Verification items for the finished model (mm, model axes). A direction names the side the tool comes from. Round coordinates to 2 decimals unless told otherwise and drop trailing zeros. Loops run counter-clockwise (first coordinate to the right, second up) from the corner with the lowest first, then second, coordinate; pieces in that order, holes last. Notation, with made-up numbers: (49, 37) -> (60, 37) arc R35 cw to (60, 73) -> close; hole circle Ø9 at (-29, 16). An arc over 180 degrees is marked (long way). Write item = value, one per line.
```python
from build123d import *

# Parameters (mm, degrees)
SKETCH_1_W             = 70
SKETCH_1_H             = 43
EXTRUDE_1_DEPTH        = 10
SKETCH_8_W             = 24.88
SKETCH_8_H             = 5
CUT_EXTRUDE_4_DEPTH    = 57.338264084
EXTRUDE_1_2_DEPTH      = 5
EXTRUDE_1_2_DEPTH_BACK = 2
SKETCH_11_R            = 20.45
SKETCH_11_R_2          = 12.45
CUT_EXTRUDE_6_DEPTH    = 5
CUT_EXTRUDE_7_DEPTH    = 5
SKETCH_16_W            = 5.88
SKETCH_16_H            = 11
CUT_EXTRUDE_8_DEPTH    = 5
SKETCH_17_W            = 5.88
SKETCH_17_H            = 8.352111755
CUT_EXTRUDE_9_DEPTH    = 5
CUT_EXTRUDE_10_DEPTH   = 5
CUT_EXTRUDE_11_DEPTH   = 5
SKETCH_21_R            = 3
CUT_EXTRUDE_12_DEPTH   = 43.275879648
SKETCH_22_R            = 3
CUT_EXTRUDE_13_DEPTH   = 43.275879648
SKETCH_24_R            = 3.51
CUT_EXTRUDE_15_DEPTH   = 7
SKETCH_27_W            = 5.88
SKETCH_27_H            = 8.139673367
CUT_EXTRUDE_16_DEPTH   = 7
SKETCH_31_W            = 6.88
SKETCH_31_H            = 8.484679277
CUT_EXTRUDE_21_DEPTH   = 14.5
CUT_EXTRUDE_22_DEPTH   = 42.379342672
CUT_EXTRUDE_23_DEPTH   = 42.379342672
CUT_EXTRUDE_24_DEPTH   = 42.379342672
CUT_EXTRUDE_25_DEPTH   = 14.5
CUT_EXTRUDE_26_DEPTH   = 14.5
CUT_EXTRUDE_27_DEPTH   = 14.5
FILLET_1_R             = 10


with BuildPart() as part:
    # 草圖1 → Extrude 1 (new body)
    with BuildSketch(Plane(origin=(0, 0, 0), x_dir=(1, 0, 0), z_dir=(0, 1, 0))):
        Rectangle(SKETCH_1_W, SKETCH_1_H)
    extrude(amount=EXTRUDE_1_DEPTH)

    # 草圖8 → 除料-伸長4 (cut, through all)
    with BuildSketch(Plane.XY.offset(21.5)):
        with Locations((0.06, 7.5)):
            Rectangle(SKETCH_8_W, SKETCH_8_H)
    extrude(amount=-CUT_EXTRUDE_4_DEPTH, mode=Mode.SUBTRACT)

    # 草圖11 → Extrude 1 2 (add, two sides: drawn at the far end of the back side and taken through both)
    with BuildSketch(Plane(origin=(0, 5, 0), x_dir=(1, 0, 0), z_dir=(0, 1, 0)).offset(-EXTRUDE_1_2_DEPTH_BACK)):
        with Locations((0.06, 0)):
            Circle(SKETCH_11_R)
        with Locations((0.06, 0)):
            Circle(SKETCH_11_R_2, mode=Mode.SUBTRACT)
    extrude(amount=EXTRUDE_1_2_DEPTH + EXTRUDE_1_2_DEPTH_BACK)

    # 草圖14 → 除料-伸長6 (cut)
    with BuildSketch(Plane(origin=(0, 5, 0), x_dir=(1, 0, 0), z_dir=(0, 1, 0))):
        Polygon((0.06, -20.45), (12.5, -20.45), (12.5, -21.5), (-12.38, -21.5), (-12.38, -20.45), align=None)
    extrude(amount=-CUT_EXTRUDE_6_DEPTH, mode=Mode.SUBTRACT)

    # 草圖15 → 除料-伸長7 (cut)
    with BuildSketch(Plane(origin=(0, 5, 0), x_dir=(1, 0, 0), z_dir=(0, 1, 0))):
        Polygon((0.06, 20.45), (12.5, 20.45), (12.5, 21.5), (-12.38, 21.5), (-12.38, 20.45), align=None)
    extrude(amount=-CUT_EXTRUDE_7_DEPTH, mode=Mode.SUBTRACT)

    # 草圖16 → 除料-伸長8 (cut)
    with BuildSketch(Plane(origin=(0, 10, 0), x_dir=(1, 0, 0), z_dir=(0, 1, 0))):
        with Locations((0.06, 17.597888245)):
            Rectangle(SKETCH_16_W, SKETCH_16_H)
    extrude(amount=-CUT_EXTRUDE_8_DEPTH, mode=Mode.SUBTRACT)

    # 草圖17 → 除料-伸長9 (cut)
    with BuildSketch(Plane(origin=(0, 10, 0), x_dir=(1, 0, 0), z_dir=(0, 1, 0))):
        with Locations((0.06, -16.273944123)):
            Rectangle(SKETCH_17_W, SKETCH_17_H)
    extrude(amount=-CUT_EXTRUDE_9_DEPTH, mode=Mode.SUBTRACT)

    # 草圖19 → 除料-伸長10 (cut)
    with BuildSketch(Plane(origin=(0, 5, 0), x_dir=(1, 0, 0), z_dir=(0, 1, 0))):
        Polygon((-2.88, 20.237561612), (-2.88, 20.45), (2.98755849, 20.45), (3, 20.237561612), align=None)
    extrude(amount=-CUT_EXTRUDE_10_DEPTH, mode=Mode.SUBTRACT)

    # 草圖20 → 除料-伸長11 (cut)
    with BuildSketch(Plane(origin=(0, 5, 0), x_dir=(1, 0, 0), z_dir=(0, 1, 0))):
        Polygon((3, -20.237561612), (3, -20.45), (-2.887827835, -20.45), (-2.88, -20.237561612), align=None)
    extrude(amount=-CUT_EXTRUDE_11_DEPTH, mode=Mode.SUBTRACT)

    # 草圖21 → 除料-伸長12 (cut, through all)
    with BuildSketch(Plane(origin=(0, 10, 0), x_dir=(1, 0, 0), z_dir=(0, 1, 0))):
        with Locations(Location((-25, 11.5, 0), (0, 0, 270))):
            Circle(SKETCH_21_R)
    extrude(amount=-CUT_EXTRUDE_12_DEPTH, mode=Mode.SUBTRACT)

    # 草圖22 → 除料-伸長13 (cut, through all)
    with BuildSketch(Plane(origin=(0, 10, 0), x_dir=(1, 0, 0), z_dir=(0, 1, 0))):
        with Locations(Location((25, 11.5, 0), (0, 0, 270))):
            Circle(SKETCH_22_R)
    extrude(amount=-CUT_EXTRUDE_13_DEPTH, mode=Mode.SUBTRACT)

    # 草圖24 → 除料-伸長15 (cut)
    with BuildSketch(Plane(origin=(0, 5, 0), x_dir=(1, 0, 0), z_dir=(0, 1, 0))):
        with Locations((0, -12.216230782)):
            Circle(SKETCH_24_R)
    extrude(amount=CUT_EXTRUDE_15_DEPTH, mode=Mode.SUBTRACT)

    # 草圖27 → 除料-伸長16 (cut)
    with BuildSketch(Plane(origin=(0, 5, 0), x_dir=(1, 0, 0), z_dir=(0, 1, 0))):
        with Locations((0.06, 16.167724929)):
            Rectangle(SKETCH_27_W, SKETCH_27_H)
    extrude(amount=-CUT_EXTRUDE_16_DEPTH, mode=Mode.SUBTRACT)

    # 草圖31 → 除料-伸長21 (cut)
    with BuildSketch(Plane(origin=(0, 10, 0), x_dir=(1, 0, 0), z_dir=(0, 1, 0))):
        with Locations((0.06, 16.207660362)):
            Rectangle(SKETCH_31_W, SKETCH_31_H)
    extrude(amount=-CUT_EXTRUDE_21_DEPTH, mode=Mode.SUBTRACT)

    # 草圖32 → 除料-伸長22 (cut, through all)
    with BuildSketch(Plane(origin=(0, 5, 0), x_dir=(1, 0, 0), z_dir=(0, 1, 0))):
        Polygon((12.5, 20.45), (12.5, 16.231109019), (10.42274151, 17.629976982), (8.239234926, 18.743068479), (5.957708545, 19.581101448), (3.5, 20.158593701), (3.5, 20.45), align=None)
    extrude(amount=-CUT_EXTRUDE_22_DEPTH, mode=Mode.SUBTRACT)

    # 草圖33 → 除料-伸長23 (cut, through all)
    with BuildSketch(Plane(origin=(0, 5, 0), x_dir=(1, 0, 0), z_dir=(0, 1, 0))):
        Polygon((-12.38, 16.231109019), (-12.38, 20.45), (-3.38, 20.45), (-3.38, 20.158593701), (-5.787343839, 19.596200398), (-8.119234926, 18.743068479), (-10.338150934, 17.609115741), align=None)
    extrude(amount=-CUT_EXTRUDE_23_DEPTH, mode=Mode.SUBTRACT)

    # 草圖34 → 除料-伸長24 (cut, through all)
    with BuildSketch(Plane(origin=(0, 5, 0), x_dir=(1, 0, 0), z_dir=(0, 1, 0))):
        Polygon((-12.38, -20.45), (-12.38, -16.231109019), (-10.215137429, -17.681177869), (-7.886635489, -18.842862957), (-5.420645085, -19.701904209), (-2.88, -20.237561612), (-2.887827835, -20.45), align=None)
    extrude(amount=-CUT_EXTRUDE_24_DEPTH, mode=Mode.SUBTRACT)

    # 草圖35 → 除料-伸長25 (cut)
    with BuildSketch(Plane(origin=(0, 5, 0), x_dir=(1, 0, 0), z_dir=(0, 1, 0))):
        Polygon((3, -20.237561612), (3, -20.45), (12.5, -20.45), (12.5, -16.231109019), (11.802562641, -16.742602026), (10.376101904, -17.657308444), (8.006635489, -18.842862957), (5.650656404, -19.670970006), align=None)
    extrude(amount=-CUT_EXTRUDE_25_DEPTH, mode=Mode.SUBTRACT)

    # 草圖37 → 除料-伸長26 (cut)
    with BuildSketch(Plane(origin=(0, 10, 0), x_dir=(1, 0, 0), z_dir=(0, 1, 0))):
        Polygon((-35, -21.5), (-12.38, -21.5), (-12.38, -16.231109019), (-35, 4.72072635), align=None)
    extrude(amount=-CUT_EXTRUDE_26_DEPTH, mode=Mode.SUBTRACT)

    # 草圖38 → 除料-伸長27 (cut)
    with BuildSketch(Plane(origin=(0, 10, 0), x_dir=(1, 0, 0), z_dir=(0, 1, 0))):
        Polygon((35, 4.72072635), (35, -21.5), (12.5, -21.5), (12.5, -16.231109019), align=None)
    extrude(amount=-CUT_EXTRUDE_27_DEPTH, mode=Mode.SUBTRACT)

    # 圓角1
    fillet_1_edges = [part.edges().sort_by_distance(p)[0] for p in [
        (-35, 5, -4.72072635),
        (35, 5, -4.72072635),
    ]]
    fillet(fillet_1_edges, radius=FILLET_1_R)


solid = part.part
```
(1) Sectioned sample at A-A, the plane y = 7.25. Record the cut outline in (x, z), and give its area (3 significant figures).
Filled sheet:
outline = (-35, -21.5) -> (-12.38, -21.5) -> (-12.38, -16.23) arc R20.45 ccw to (-3.38, -20.16) -> (-3.38, -11.97) arc R12.45 cw to (-12.38, -0.5) -> (-12.38, 0.5) arc R12.45 cw to (-3.5, 11.93) arc R3.51 cw to (-2.88, 14.22) -> (-2.88, 20.24) arc R20.45 ccw to (-12.38, 16.23) -> (-31.8, -1.75) arc R10 ccw to (-35, -9.09) -> close; (3, 14.04) arc R3.51 cw to (3.5, 11.97) arc R12.45 cw to (12.5, 0.5) -> (12.5, -0.5) arc R12.45 cw to (3.5, -11.97) -> (3.5, -20.16) arc R20.45 ccw to (12.5, -16.23) -> (12.5, -21.5) -> (35, -21.5) -> (35, -9.07) arc R10 ccw to (31.81, -1.75) -> (12.5, 16.23) arc R20.45 ccw to (3, 20.24) -> close; hole circle Ø6 at (-25, -11.5); hole circle Ø6 at (25, -11.5)
area = 1,530 mm2
(2) Set-up check for faces 4 (the face through (-9.67, 7.46, -7.77)), 5 (the face through (-2.88, 8, 17)), 6 (the face through (0, 3, -11.965)): record each of +Z, -Z, +X, -X, +Y, -Y from which the full face is reachable in a straight line by a thin tool's end or side.
Filled sheet:
face_4 = +Y
face_5 = +Z, -Z, +Y
face_6 = -Z, +Y, -Y
(3) Sectioned sample at B-B, the plane x = 25. Record the cut outline in (y, z).
Filled sheet:
outline = (0, -21.5) -> (10, -21.5) -> (10, -14.5) -> (0, -14.5) -> close; (0, -8.5) -> (10, -8.5) -> (10, 4.59) -> (0, 4.59) -> close
(4) Material ranges on probe 1 along X at (y, z) = (2.5, -11.5); probe 2 along X at (y, z) = (6.5, -11.5); probe 3 along Y at (x, z) = (-5.5, 4.5), recorded low to high. Write a range as from..to.
Filled sheet:
probe_1 = -35..-28, -22..22, 28..35
probe_2 = -35..-28, -22..-4.71, 4.83..22, 28..35
probe_3 = 0..5
(5) Sectioned sample at D-D, the plane y = 1. Count the separate pieces of the cut face and the enclosed holes in it, and give its area (3 significant figures).
Filled sheet:
separate_pieces = 1
enclosed_holes = 2
area = 2,060 mm2
(6) Draft check along Z on faces 1 (the face through (7.94, 7.46, 18.87)), 2 (the face through (-3.393, 7.465, 13.114)), 3 (the face through (7.114, 2.535, -19.156)). Enter one of: released by +Z, released by -Z, zero draft, split by the parting line, or undercut.
Filled sheet:
face_1 = released by +Z
face_2 = undercut
face_3 = released by -Z
(7) Sectioned sample at C-C, the plane z = -10.5. Record the cut outline in (x, y).
Filled sheet:
outline = (-35, 0) -> (-27.83, 0) -> (-27.83, 10) -> (-35, 10) -> close; (-22.17, 0) -> (22.17, 0) -> (22.17, 10) -> (6.75, 10) -> (6.75, 5) -> (-6.63, 5) -> (-6.63, 10) -> (-22.17, 10) -> close; (27.83, 0) -> (35, 0) -> (35, 10) -> (27.83, 10) -> close
(8) Go/stop test with flat-tipped pins: pin 1 Ø2 at (y, z) = (2, 8) entering from -X; pin 2 Ø2.5 at (y, z) = (7.5, 18) entering from -X; pin 3 Ø2.5 at (y, z) = (8.5, 18.5) entering from +X; pin 4 Ø0.7 at (x, z) = (7, 19) entering from -Y. Record where each tip stops, or that it passes through.
Filled sheet:
pin_1 = -22.35
pin_2 = -11.67
pin_3 = 11.04
pin_4 = 0
